Build history of the part. All positions in model axes, mm. Face numbers are marked on the shaded views. Round coordinates to 2 decimals unless told otherwise and drop trailing zeros. Loops run counter-clockwise (first coordinate to the right, second up) from the corner with the lowest first, then second, coordinate; pieces in that order, holes last.
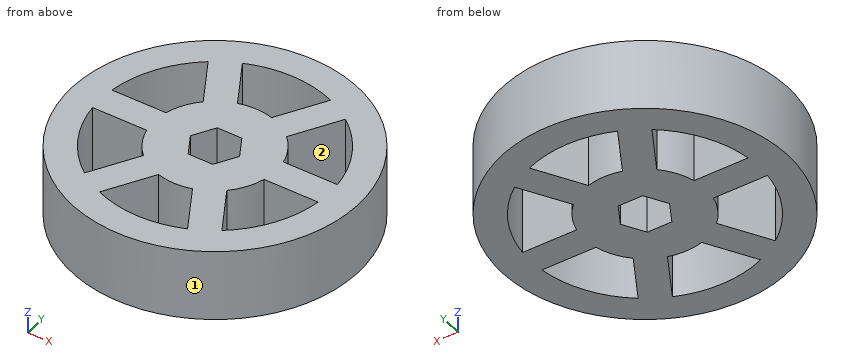
Autodesk Inventor part; units mm, degrees
ref_plane "YZ Plane" through (0, 0, 0) normal (1, 0, 0) x (0, 1, 0)
ref_plane "XZ Plane" through (0, 0, 0) normal (0, 1, 0) x (-1, 0, 0)
ref_plane "XY Plane" through (0, 0, 0) normal (0, 0, 1) x (1, 0, 0)
sketch "Sketch1" plane through (0, 0, 0) normal (0, 0, 1) x (1, 0, 0)
  line L0 (2.1997, 3.81) -> (4.3994, 0)
  line L1 (4.3994, 0) -> (2.1997, -3.81)
  line L2 (2.1997, -3.81) -> (-2.1997, -3.81)
  line L3 (-2.1997, -3.81) -> (-4.3994, 0)
  line L4 (-4.3994, 0) -> (-2.1997, 3.81)
  line L5 (-2.1997, 3.81) -> (2.1997, 3.81)
  line L6 (0, 0) -> (1.743, 0)
  circle A0 centre (0, 0) radius 10.795
  circle A1 centre (0, 0) radius 25.4
  circle A2 centre (0, 0) radius 20.32
  line L7 (-4.3994, 0) -> (-20.32, 0)
  line L8 (-2.1997, 3.81) -> (-10.16, 17.5976)
  line L9 (2.1997, 3.81) -> (10.16, 17.5976)
  line L10 (4.3994, 0) -> (20.32, 0)
  line L11 (2.1997, -3.81) -> (10.16, -17.5976)
  line L12 (-2.1997, -3.81) -> (-10.16, -17.5976)
  line L13 (-2.9329, 2.54) -> (-20.1606, 2.54)
  line L14 (-2.9329, -2.54) -> (-20.1606, -2.54)
  line L15 (-3.6662, -1.27) -> (-12.28, -16.1896)
  line L16 (0.7332, -3.81) -> (-7.8806, -18.7296)
  line L17 (-0.7332, -3.81) -> (7.8806, -18.7296)
  line L18 (3.6662, -1.27) -> (12.28, -16.1896)
  line L19 (2.9329, 2.54) -> (20.1606, 2.54)
  line L20 (2.9329, -2.54) -> (20.1606, -2.54)
  line L21 (-7.4457, 7.8163) -> (-12.28, 16.1896)
  line L22 (-3.0463, 10.3563) -> (-7.8806, 18.7296)
  line L23 (-0.7332, 3.81) -> (7.8806, 18.7296)
  line L24 (3.6662, 1.27) -> (12.28, 16.1896)
  dimension "d0" = 7.62
  dimension "d1" = 21.59
  dimension "d2" = 50.8
  dimension "d3" = 5.08
  dimension "d4" = 120
  dimension "d5" = 120
  dimension "d6" = 120
  dimension "d7" = 120
  dimension "d8" = 5.08
  dimension "d9" = 2.54
  dimension "d10" = 5.08
  dimension "d11" = 2.54
  dimension "d13" = 2.54
  dimension "d14" = 5.08
  dimension "d15" = 5.08
  dimension "d17" = 2.54
  dimension "d18" = 2.54
  dimension "d19" = 2.54
  dimension "d20" = 5.08
  dimension "d21" = 2.54
extrude "Extrusion1" add sketch "Sketch1" along normal blind 12.7 contours L9 A0 L24 L19 L0 | L5 L23 A0 L9 | L19 L24 L0 | L5 L8 A0 L23 | L9 A2 L24 A0 | A0 L23 A2 L9 | L24 L19 A0 L10 L0 | L24 A0 L19 | L4 L13 A0 L8 | L10 A0 L20 L18 L1 | L19 A2 L10 A0 | L4 L7 A0 L13 | L8 A2 L22 A0 | A0 L21 A2 L8 | L18 L20 L1 | L10 A2 L20 A0 | L3 L15 L14 A0 L7 | A0 L7 A2 L13 | L20 L18 A0 L11 L1 | L20 A0 L18 | L3 L14 L15 | A0 L14 A2 L7 | L11 A0 L17 L16 L2 | L18 A2 L11 A0 | L3 L12 A0 L15 L14 | L15 A0 L14 | L16 L17 L2 | L11 A2 L17 A0 | L2 L17 L16 A0 L12 | A0 L12 A2 L15 | L17 A0 L16 | A0 L16 A2 L12 | A1
equation "\"d5\" = d4"
equation "\"d6\" = d4"
equation "\"d7\" = d4"
properties part number "RobotArm Wheel2"
(1) Slice it at A-A on x = 0. List the corners of the cut face in (y, z) (3 decimals), plus the area to 3 significant figures.
Responses:
outline: (-25.4, 0) - (-20.32, 0) - (-20.32, 12.7) - (-25.4, 12.7) - close; (-10.795, 0) - (-3.81, 0) - (-3.81, 12.7) - (-10.795, 12.7) - close; (3.81, 0) - (10.795, 0) - (10.795, 12.7) - (3.81, 12.7) - close; (20.32, 0) - (25.4, 0) - (25.4, 12.7) - (20.32, 12.7) - close
area: 306 mm2
(2) Slice it at D-D on y = -17. List the corners of the cut face in (x, z).
Responses:
outline: (-18.87, 0) - (-6.88, 0) - (-6.88, 12.7) - (-18.87, 12.7) - close; (6.88, 0) - (18.87, 0) - (18.87, 12.7) - (6.88, 12.7) - close
(3) Pin check, flat tips, straight feed: P1, Ø4, axis at x = -15.5, z = 8.5, coming from the -Y side; P2, Ø7.5, axis at x = 17.5, z = 5, coming from the +Y side; P3, Ø7.5, axis at x = 13.5, z = 7.5, coming from the -Y side. Stop position of each tip, or through.
Responses:
P1: stops at y = -21.52
P2: stops at y = 21.36
P3: stops at y = -23.45
(4) Probe line 1 (Y direction, x = -0.5, z = 2.5); line 2 (Y direction, x = 14, z = 1); line 3 (Y direction, x = 15.5, z = 1.5). List the from-to ranges inside material, lowest first.
Responses:
line 1: y = -25.4 to -20.31, -10.78 to -3.81, 3.81 to 10.78, 20.31 to 25.4
line 2: y = -21.19 to -14.73, -2.54 to 2.54, 14.73 to 21.19
line 3: y = -20.12 to -13.14, -2.54 to 2.54, 13.14 to 20.12
(5) Slice it at C-C on z = 4.25. Count the separate pieces of the cut face and the enclosed holes in it, plus the area to 3 significant figures.
Responses:
separate pieces: 1
enclosed holes: 7
area: 1,340 mm2
(6) Pull direction X, two halves, no side cores. Call the marked faces 1 and 2: +X half, -X half, draft (parallel to the pull), parting line (faces both ways), or undercut.
Responses:
face 1: parting line
face 2: undercut
(7) Slice it at B-B on x = -13. List the corners of the cut face in (y, z), plus the area to 3 significant figures.
Responses:
outline: (-21.82, 0) - (-15.62, 0) - (-15.62, 12.7) - (-21.82, 12.7) - close; (-2.54, 0) - (2.54, 0) - (2.54, 12.7) - (-2.54, 12.7) - close; (15.62, 0) - (21.82, 0) - (21.82, 12.7) - (15.62, 12.7) - close
area: 222 mm2
